from build123d import *

# Parameters (mm, degrees)
BOSS_EXTRUDE1_DEPTH = 18
SKETCH2_W           = 3
SKETCH2_H           = 2
CUT_EXTRUDE1_DEPTH  = 185.274252135
SKETCH3_W           = 183
SKETCH3_H           = 18
CUT_EXTRUDE2_DEPTH  = 12


with BuildPart() as part:
    # Sketch1 → Boss-Extrude1 (new body)
    with BuildSketch(Plane(origin=(0, 0, 0), x_dir=(1, 0, 0), z_dir=(0, 1, 0))):
        Polygon((183, 0), (0, 0), (12, 12), (183, 12), align=None)
    boss_extrude1 = extrude(amount=BOSS_EXTRUDE1_DEPTH)

    # Sketch2 → Cut-Extrude1 (cut, symmetric)
    with BuildSketch(Plane(origin=(183, 0, 0), x_dir=(0, 0, -1), z_dir=(1, 0, 0))):
        with Locations((10.5, 14)):
            Rectangle(SKETCH2_W, SKETCH2_H)
    cut_extrude1 = extrude(amount=CUT_EXTRUDE1_DEPTH, both=True, mode=Mode.SUBTRACT)

    # Mirror2: Boss-Extrude1, Cut-Extrude1 across plane
    add(boss_extrude1.mirror(Plane(origin=(0, 18, -12), x_dir=(1, 0, 0), z_dir=(0, 0, -1))))
    add(cut_extrude1.mirror(Plane(origin=(0, 18, -12), x_dir=(1, 0, 0), z_dir=(0, 0, -1))), mode=Mode.SUBTRACT)

    # Sketch3 → Cut-Extrude2 (cut)
    with BuildSketch(Plane.XY):
        with Locations((91.5, 9)):
            Rectangle(SKETCH3_W, SKETCH3_H)
    extrude(amount=-CUT_EXTRUDE2_DEPTH, mode=Mode.SUBTRACT)


solid = part.part
The listing builds one solid part. Answer for the finished solid, in the listing's coordinates (mm). Coordinates: 2 decimals unless noted, no trailing zeros. Loops run counter-clockwise (first coordinate to the right, second up) from the corner with the lowest first, then second, coordinate; pieces in that order, holes last. Notation, with made-up numbers: (89.25, 25.5) -> (129.25, 25.5) arc R34 ccw to (129.25, 55.5) -> close; hole circle Ø8 at (48.25, 77.25). An arc over 180 degrees is marked (long way). Write item = value, one per line. Start each with the question number.
1) Given pin 1 Ø5 at (y, z) = (2, -19) entering from -X; pin 2 Ø1 at (x, y) = (109.5, 14) entering from +Z; pin 3 Ø4 at (x, z) = (148, -17.5) entering from -Y; pin 4 Ø6 at (y, z) = (2, -14) entering from -X, each flat-ended and moving along its own axis, determine where each tip first touches the part or whether it passes through.
2) The mould has two halves that part along Y. Classify faces 1 (the face through (96, 7, -12)), 2 (the face through (97, 15, -13)), 3 (the face through (97, 13, -13)), 4 (the face through (93, 18, -18)): released by +Y, released by -Y, zero draft, split by the parting line, or undercut.
3) A cutting plane is placed at D-D (z = -21). Give the vertices of the cut face in (x, y).
4) A cutting plane is placed at C-C (y = 10). Give the vertices of the cut face in (x, z), then the cut area to 3 significant figures.
5) Straight lines are drawn through the part: line 1 (Y direction, x = 96.5, z = -14.75); line 2 (Z direction, x = 105.5, y = 14); line 3 (X direction, y = 9, z = -13.5). For each, find the intervals that lie inside material, in ascending order. Write a range as from..to.
6) A cutting plane is placed at B-B (x = 91). Give the vertices of the cut face in (y, z), then the cut area to 3 significant figures.
7) A cutting plane is placed at A-A (z = -13.5). Give the vertices of the cut face in (x, y), then the cut area to 3 significant figures.
Responses:
q1.pin_1 = 2.5
q1.pin_2 = -15
q1.pin_3 = 0
q1.pin_4 = 7
q2.face_1 = zero draft
q2.face_2 = undercut
q2.face_3 = undercut
q2.face_4 = released by +Y
q3.outline = (3, 0) -> (183, 0) -> (183, 18) -> (3, 18) -> close
q4.outline = (0, -24) -> (183, -24) -> (183, -12) -> (12, -12) -> close
q4.area = 2,120 mm²
q5.line_1 = 0..13, 15..18
q5.line_2 = -24..-15
q5.line_3 = 10.5..183
q6.outline = (0, -24) -> (18, -24) -> (18, -12) -> (15, -12) -> (15, -15) -> (13, -15) -> (13, -12) -> (0, -12) -> close
q6.area = 210 mm²
q7.outline = (10.5, 0) -> (183, 0) -> (183, 13) -> (10.5, 13) -> close; (10.5, 15) -> (183, 15) -> (183, 18) -> (10.5, 18) -> close
q7.area = 2,760 mm²
